Verification items for the finished model (mm, model axes). Round coordinates to 2 decimals unless told otherwise and drop trailing zeros. Loops run counter-clockwise (first coordinate to the right, second up) from the corner with the lowest first, then second, coordinate; pieces in that order, holes last. Notation, with made-up numbers: (68, -27.75) -> (85, -27.75) arc R27 ccw to (85, -6.75) -> close; hole circle Ø2 at (71.25, -36). An arc over 180 degrees is marked (long way). Write item = value, one per line.
```python
from build123d import *

# Parameters (mm, degrees)
SKETCH_1_W          = 297
SKETCH_1_H          = 444
EXTRUDE_1_DEPTH     = 47
SKETCH_2_W          = 255
SKETCH_2_H          = 408
CUT_EXTRUDE_1_DEPTH = 2
SKETCH_3_W          = 74
SKETCH_3_H          = 444
CUT_EXTRUDE_2_DEPTH = 24.736842105


with BuildPart() as part:
    # 草圖1 → 填料-伸長1 (new body)
    with BuildSketch(Plane(origin=(0, 0, 0), x_dir=(1, 0, 0), z_dir=(0, 1, 0))):
        Rectangle(SKETCH_1_W, SKETCH_1_H)
    extrude(amount=EXTRUDE_1_DEPTH)

    # 草圖2 → 除料-伸長1 (cut)
    with BuildSketch(Plane(origin=(0, 47, 0), x_dir=(1, 0, 0), z_dir=(0, 1, 0))):
        Rectangle(SKETCH_2_W, SKETCH_2_H)
    extrude(amount=-CUT_EXTRUDE_1_DEPTH, mode=Mode.SUBTRACT)

    # 草圖3 → 除料-伸長2 (cut)
    with BuildSketch(Plane.XZ):
        with Locations((-111.5, 0)):
            Rectangle(SKETCH_3_W, SKETCH_3_H)
    extrude(amount=-CUT_EXTRUDE_2_DEPTH, mode=Mode.SUBTRACT)


solid = part.part
```
(1) Draft check along X on faces 1 (the face through (-2, 45, -3)), 2 (the face through (-112, 24.737, 3)), 3 (the face through (148.5, 23, 3)), 4 (the face through (-74.5, 12, -3)). Enter one of: released by +X, released by -X, zero draft, split by the parting line, or undercut.
Filled sheet:
face_1 = undercut
face_2 = zero draft
face_3 = released by +X
face_4 = released by -X
(2) Sectioned sample at D-D, the plane y = 8.5. Record the cut outline in (x, z).
Filled sheet:
outline = (-74.5, -222) -> (148.5, -222) -> (148.5, 222) -> (-74.5, 222) -> close
(3) Material ranges on probe 1 along Y at (x, z) = (15, -154); probe 2 along Y at (x, z) = (-133, 16); probe 3 along X at (y, z) = (19.5, -147), recorded low to high. Write a range as from..to.
Filled sheet:
probe_1 = 0..45
probe_2 = 24.74..47
probe_3 = -74.5..148.5
(4) Sectioned sample at B-B, the plane x = -56.5. Record the cut outline in (y, z).
Filled sheet:
outline = (0, -222) -> (47, -222) -> (47, -204) -> (45, -204) -> (45, 204) -> (47, 204) -> (47, 222) -> (0, 222) -> close
(5) Go/stop test with flat-tipped pins: pin 1 Ø5 at (x, z) = (-15, 120.5) entering from +Y; pin 2 Ø6 at (y, z) = (5, 4) entering from -X; pin 3 Ø22 at (x, z) = (-130, -6) entering from -Y. Record where each tip stops, or that it passes through.
Filled sheet:
pin_1 = 45
pin_2 = -74.5
pin_3 = 24.74
(6) Sectioned sample at A-A, the plane z = -19. Record the cut outline in (x, y).
Filled sheet:
outline = (-148.5, 24.74) -> (-74.5, 24.74) -> (-74.5, 0) -> (148.5, 0) -> (148.5, 47) -> (127.5, 47) -> (127.5, 45) -> (-127.5, 45) -> (-127.5, 47) -> (-148.5, 47) -> close
(7) Sectioned sample at C-C, the plane x = -119.5. Record the cut outline in (y, z), and give its area (3 significant figures).
Filled sheet:
outline = (24.74, -222) -> (47, -222) -> (47, -204) -> (45, -204) -> (45, 204) -> (47, 204) -> (47, 222) -> (24.74, 222) -> close
area = 9,070 mm2
